from build123d import *

# Parameters (mm, degrees)
BOX_W     = 45
BOX_H     = 25
BOX_DEPTH = 12.5


with BuildPart() as sphere001:
    # Sphere001 → Sphere001 (revolve)
    with BuildSketch(Plane(origin=(30, 0, 0), x_dir=(1, 0, 0), z_dir=(0, -1, 0))):
        with BuildLine():
            ThreePointArc((0, -10), (10, 0), (0, 10))
            Line((0, 10), (0, -10))
        make_face()
    revolve(axis=Axis((30, 0, 0), (0, 0, 1)))


with BuildPart() as cube:
    # Box → Box (new body)
    with BuildSketch(Plane(origin=(-2.5, -12.5, -12.5), x_dir=(1, 0, 0), z_dir=(0, 0, 1))):
        with Locations((22.5, 12.5)):
            Rectangle(BOX_W, BOX_H)
    extrude(amount=BOX_DEPTH)


with BuildPart() as cut:
    # Sphere → Sphere (revolve)
    with BuildSketch(Plane(origin=(10, 0, 0), x_dir=(1, 0, 0), z_dir=(0, -1, 0))):
        with BuildLine():
            ThreePointArc((0, -10), (10, 0), (0, 10))
            Line((0, 10), (0, -10))
        make_face()
    revolve(axis=Axis((10, 0, 0), (0, 0, 1)))

    # Fusion: union Cube
    add(cube.part)

    # Cut: cut Sphere001
    add(sphere001.part, mode=Mode.SUBTRACT)


solid = cut.part
Model file for the job. Use its own axes, mm. A direction names the side the tool comes from. Give positions to 0.01 mm unless a question says otherwise; leave off trailing zeros. Write each loop counter-clockwise with the first axis right and the second up, starting at its lowest first coordinate (ties: lowest second). Pieces come first, ordered by that corner, then holes. Notation, with made-up numbers: (88.5, -8.75) - (130.5, -8.75) arc R12 cw to (130.5, -0.75) - close; hole circle Ø10 at (49.5, -20.5). An arc over 180 degrees is marked (long way). Answer as CSV lines item,"result".
1. Pin check, flat tips, straight feed: pin 1 (2 mm diameter, centred on x = 3, z = 4, fed in from +Y); pin 2 (4 mm diameter, centred on x = 25, y = -3, fed in from +Z); pin 3 (2 mm diameter, centred on y = -4.5, z = 3.5, fed in from -X). Stop position of each tip, or through.
Responses:
pin 1,"stops at y = 7.08"
pin 2,"stops at z = -6.22"
pin 3,"stops at x = 1.17"
2. Band-saw the part on D-D (z = -5). Write the cut outline in (x, y), and give its area (3 significant figures).
Responses:
outline,"(-2.5, -12.5) - (42.5, -12.5) - (42.5, 12.5) - (-2.5, 12.5) - close; hole circle Ø17.32 at (30, 0)"
area,"889 mm2"
3. Band-saw the part on C-C (y = -3.5). Write the cut outline in (x, z) (1 decimal), and give its area (4 significant figures).
Responses:
outline,"(-2.5, -12.5) - (42.5, -12.5) - (42.5, 0) - (39.4, 0) arc R9.4 cw to (20.6, 0) - (19.4, 0) arc R9.4 ccw to (0.6, 0) - (-2.5, 0) - close"
area,"562.5 mm2"
4. Band-saw the part on A-A (x = 16). Write the cut outline in (y, z), and give its area (3 significant figures).
Responses:
outline,"(-12.5, -12.5) - (12.5, -12.5) - (12.5, 0) - (8, 0) arc R8 ccw to (-8, 0) - (-12.5, 0) - close"
area,"413 mm2"
5. Drill centre lines: L1, parallel to Z at x = 38.5, y = -11; L2, parallel to Y at x = 23, z = -5.75; L3, parallel to X at y = -4, z = -3.75. Where is each one in solid material? Low to high. Write a range as [from, to].
Responses:
L1,"z = [-12.5, 0]"
L2,"y = [-12.5, -4.24], [4.24, 12.5]"
L3,"x = [-2.5, 21.64], [38.36, 42.5]"
6. Band-saw the part on B-B (z = -0.5). Write the cut outline in (x, y), and give its area (3 significant figures).
Responses:
outline,"(-2.5, -12.5) - (42.5, -12.5) - (42.5, 12.5) - (-2.5, 12.5) - close; hole circle Ø19.97 at (30, 0)"
area,"812 mm2"
7. 3-axis set-ups, long thin cutter, end or side, ignore diameter. For faces 1 (the face through (20, 3, 0)), 2 (the face through (20, -12.5, -6)): which of +Z, -Z, +X, -X, +Y, -Y reach the whole face in a straight line?
Responses:
face 1,"+Z"
face 2,"+Z, -Z, +X, -X, -Y"
